The listing builds one solid part. Answer for the finished solid, in the listing's coordinates (mm). Face numbers are marked on the shaded views. A direction names the side the tool comes from. Give positions to 0.01 mm unless a question says otherwise; leave off trailing zeros. Order: outer loops, then holes, each group sorted by start corner. A loop starts at its lowest first (then second) coordinate and runs counter-clockwise, first axis right, second up. Notation, with made-up numbers: (-20.5, 20) - (33.5, 20) arc R9 ccw to (33.5, 24) - close; hole circle Ø3 at (71, -5). An arc over 180 degrees is marked (long way). Use a Markdown table: item, result. Add a question column.
1) Find section B-B, the plane z = 8. Determine the outline of the cut face in (x, y), plus the area to 3 significant figures.
2) The mould has two halves that part along X. Classify the marked faces 1, 2, 3 and 4: released by +X, released by -X, zero draft, split by the parting line, or undercut.
3) Find section A-A, the plane x = 0. Determine the outline of the cut face in (y, z), plus the area to 3 significant figures.
4) Flat-ended cylindrical pins translate along their axes: pin 1 (7 mm diameter, centred on x = 27.5, z = 8, fed in from +Y); pin 2 (1 mm diameter, centred on y = 29, z = 4, fed in from -X); pin 3 (1.5 mm diameter, centred on y = 18.5, z = 9.5, fed in from +X). Find the tip coordinate at first contact, or state that the pin passes through.
5) Straight lines are drawn through the part: line 1 (X direction, y = 2.65, z = 8); line 2 (Y direction, x = 0, z = 7.25); line 3 (Z direction, x = -27.5, y = 2.45). For each, find the intervals that lie inside material, in ascending order.
6) Find section D-D, the plane x = -23. Determine the outline of the cut face in (y, z), plus the area to 3 significant figures.
7) Find section C-C, the plane x = 27.5. Determine the outline of the cut face in (y, z), plus the area to 3 significant figures.
8) For the marked faces 5 and 6, determine the directions among +Z, -Z, +X, -X, +Y, -Y from which every point of the face is accessible in a straight line to the end or side of a thin tool.
from build123d import *

# Parameters (mm, degrees)
SKETCH1_R               = 15
BOSS_EXTRUDE1_DEPTH     = 16
FILLET1_R               = 5
SKETCH2_R               = 3
CUT_EXTRUDE1_DEPTH      = 33
CUT_EXTRUDE1_DEPTH_BACK = 7
CHAMFER1_SIZE           = 2
CHAMFER1_SIZE2          = 3.5
CHAMFER2_SIZE           = 3.5
CHAMFER2_SIZE2          = 2
FILLET2_R               = 1


with BuildPart() as part:
    # Sketch1 → Boss-Extrude1 (new body)
    with BuildSketch(Plane.XY):
        with BuildLine():
            Line((-35.5, 0), (35.5, 0))
            Line((35.5, 0), (35.5, 6))
            Line((35.5, 6), (19, 6))
            Line((19, 6), (19, 19))
            ThreePointArc((19, 19), (0, 38), (-19, 19))
            Line((-19, 19), (-19, 6))
            Line((-19, 6), (-35.5, 6))
            Line((-35.5, 6), (-35.5, 0))
        make_face()
        with Locations((0, 19)):
            Circle(SKETCH1_R, mode=Mode.SUBTRACT)
    extrude(amount=BOSS_EXTRUDE1_DEPTH)

    # Fillet1
    fillet1_edges = [part.edges().sort_by_distance(p)[0] for p in [
        (35.5, 3, 0),
        (-35.5, 3, 16),
        (35.5, 3, 16),
        (-35.5, 3, 0),
    ]]
    fillet(fillet1_edges, radius=FILLET1_R)

    # Sketch2 → Cut-Extrude1 (cut, two sides)
    with BuildSketch(Plane(origin=(0, 6, 0), x_dir=(1, 0, 0), z_dir=(0, 1, 0))) as cut_extrude1_sk:
        with Locations((-27.5, -8)):
            Circle(SKETCH2_R)
        with Locations((27.5, -8)):
            Circle(SKETCH2_R)
    extrude(amount=CUT_EXTRUDE1_DEPTH, mode=Mode.SUBTRACT)
    extrude(cut_extrude1_sk.sketch, amount=-CUT_EXTRUDE1_DEPTH_BACK, mode=Mode.SUBTRACT)

    # Chamfer1
    chamfer1_edges = [part.edges().sort_by_distance(p)[0] for p in [
        (-15, 19, 16),
    ]]
    chamfer1_side = [part.faces().sort_by_distance(p)[0] for p in [
        (0, 0.718679344, 16),
    ]]
    chamfer(chamfer1_edges, length=CHAMFER1_SIZE, length2=CHAMFER1_SIZE2, reference=chamfer1_side[0])

    # Chamfer2
    chamfer2_edges = [part.edges().sort_by_distance(p)[0] for p in [
        (-15, 19, 0),
    ]]
    chamfer2_side = [part.faces().sort_by_distance(p)[0] for p in [
        (-15, 19, 6.25),
    ]]
    chamfer(chamfer2_edges, length=CHAMFER2_SIZE, length2=CHAMFER2_SIZE2, reference=chamfer2_side[0])

    # Fillet2
    fillet2_edges = [part.edges().sort_by_distance(p)[0] for p in [
        (0, 38, 0),
        (19, 12.5, 0),
        (19, 12.5, 16),
        (0, 38, 16),
        (-19, 12.5, 16),
        (-24.75, 6, 16),
        (-35.5, 6, 8),
        (24.75, 6, 0),
        (-34.035533906, 6, 14.535533906),
        (-34.035533906, 6, 1.464466094),
        (24.75, 6, 16),
        (35.5, 6, 8),
        (34.035533906, 6, 14.535533906),
        (34.035533906, 6, 1.464466094),
        (-24.75, 6, 0),
        (-19, 12.5, 0),
    ]]
    fillet(fillet2_edges, radius=FILLET2_R)


solid = part.part
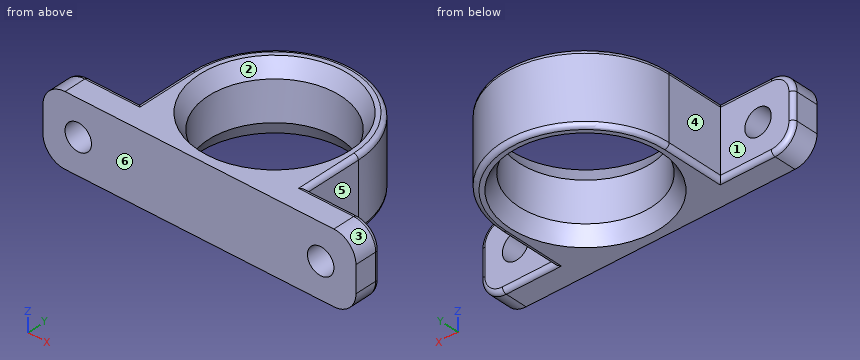
The answers:
| question | item | result |
|---|---|---|
| 1 | outline | (-35.5, 0) - (-30.5, 0) - (-30.5, 6) - (-34.5, 6) arc R1 ccw to (-35.5, 5) - close; (-24.5, 0) - (24.5, 0) - (24.5, 6) - (19, 6) - (19, 19) arc R19 ccw to (-19, 19) - (-19, 6) - (-24.5, 6) - close; (30.5, 0) - (35.5, 0) - (35.5, 5) arc R1 ccw to (34.5, 6) - (30.5, 6) - close; hole circle Ø30 at (0, 19) |
| 1 | area | 708 mm2 |
| 2 | face 1 | zero draft |
| 2 | face 2 | undercut |
| 2 | face 3 | released by +X |
| 2 | face 4 | released by -X |
| 3 | outline | (0, 0) - (2, 0) - (4, 3.5) - (4, 12.5) - (2, 16) - (0, 16) - close; (34, 3.5) - (36, 0) - (37, 0) arc R1 ccw to (38, 1) - (38, 15) arc R1 ccw to (37, 16) - (36, 16) - (34, 12.5) - close |
| 3 | area | 114 mm2 |
| 4 | pin 1 | y = 6 |
| 4 | pin 2 | x = -16.45 |
| 4 | pin 3 | x = 19 |
| 5 | line 1 | -35.5 to -30.5, -24.5 to 24.5, 30.5 to 35.5 |
| 5 | line 2 | 0 to 4, 34 to 38 |
| 5 | line 3 | 0 to 5, 11 to 16 |
| 6 | outline | (0, 0) - (5, 0) arc R1 ccw to (6, 1) - (6, 15) arc R1 ccw to (5, 16) - (0, 16) - close |
| 6 | area | 95.6 mm2 |
| 7 | outline | (0, 0) - (5, 0) arc R1 ccw to (6, 1) - (6, 5) - (0, 5) - close; (0, 11) - (6, 11) - (6, 15) arc R1 ccw to (5, 16) - (0, 16) - close |
| 7 | area | 59.6 mm2 |
| 8 | face 5 | +Z, -Z, +X, +Y |
| 8 | face 6 | +Z, -Z, +X, -X, -Y |
